from build123d import *

# Parameters (mm, degrees)
SKETCH_1_R          = 4
EXTRUDE_1_DEPTH     = 20
SKETCH_2_R          = 17
CUT_EXTRUDE_1_DEPTH = 5
CUT_EXTRUDE_START   = 15
SKETCH_2_2_R        = 17
CUT_EXTRUDE_2_DEPTH = 5


with BuildPart() as part:
    # 草图1 → 凸台-拉伸1 (new body)
    with BuildSketch(Plane.XY):
        with BuildLine():
            Line((0, 15), (75, 15))
            ThreePointArc((75, 15), (90, 0), (75, -15))
            Line((75, -15), (0, -15))
            ThreePointArc((0, -15), (-15, 0), (0, 15))
        make_face()
        Circle(SKETCH_1_R, mode=Mode.SUBTRACT)
        with Locations((75, 0)):
            Circle(SKETCH_1_R, mode=Mode.SUBTRACT)
    extrude(amount=EXTRUDE_1_DEPTH)

    # 草图2 → 切除-拉伸1 (cut)
    with BuildSketch(Plane.XY):
        Circle(SKETCH_2_R)
    extrude(amount=CUT_EXTRUDE_1_DEPTH, mode=Mode.SUBTRACT)

    # 草图2<2> → 切除-拉伸2 (cut)
    with BuildSketch(Plane.XY.offset(CUT_EXTRUDE_START)):
        Circle(SKETCH_2_2_R)
    extrude(amount=CUT_EXTRUDE_2_DEPTH, mode=Mode.SUBTRACT)


solid = part.part
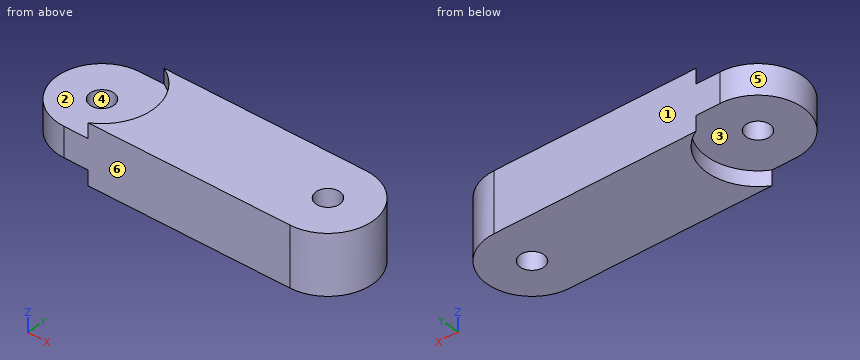
Read the model definition and answer for the solid it produces. Units are mm, in the model's axes. Face numbers are marked on the shaded views. A direction names the side the tool comes from. Give positions to 0.01 mm unless a question says otherwise; leave off trailing zeros. Loops run counter-clockwise (first coordinate to the right, second up) from the corner with the lowest first, then second, coordinate; pieces in that order, holes last. Notation, with made-up numbers: M 48,-34 L 105,-34 A15 cw 105,-5 Z; hole C 34.5,17 d5. An arc over 180 degrees is marked long. Write each question's results on one line, items separated by ' | '.
1. Section B-B on z = 3 is taken. Give the vertices of the cut face in (x, y), plus the area to 3 significant figures.
Values:
outline: M 8,-15 L 75,-15 A15 ccw 75,15 L 8,15 A17 cw Z; hole C 75,0 d8 | area: 2,120 mm^2
2. Section D-D on z = 11.75 is taken. Give the vertices of the cut face in (x, y), plus the area to 3 significant figures.
Values:
outline: M 0,-15 L 75,-15 A15 ccw 75,15 L 0,15 A15 ccw Z; hole C 0,0 d8; hole C 75,0 d8 | area: 2,860 mm^2
3. Section C-C on x = 76 is taken. Give the vertices of the cut face in (y, z).
Values:
outline: M -14.97,0 L -3.87,0 L -3.87,20 L -14.97,20 Z; M 3.87,0 L 14.97,0 L 14.97,20 L 3.87,20 Z
4. Given pin 1 (4 mm diameter, centred on x = 55.5, y = 10.5, fed in from -Z); pin 2 (9 mm diameter, centred on x = 4, y = -2, fed in from +Z); pin 3 (15 mm diameter, centred on x = -2, y = -3.5, fed in from -Z); pin 4 (8 mm diameter, centred on y = -10.5, z = 2.5, fed in from +X), each flat-ended and moving along its own axis, determine where each tip first touches the part or whether it passes through.
Values:
pin 1: stops at z = 0 | pin 2: stops at z = 15 | pin 3: stops at z = 5 | pin 4: stops at x = 88.52
5. Straight lines are drawn through the part: line 1 (Y direction, x = 75, z = 9); line 2 (Z direction, x = -9.5, y = 4); line 3 (X direction, y = 1, z = 7.5). For each, find the intervals that lie inside material, in ascending order. Write a range as [from, to].
Values:
line 1: y = [-15, -4], [4, 15] | line 2: z = [5, 15] | line 3: x = [-14.97, -3.87], [3.87, 71.13], [78.87, 89.97]
6. Section A-A on y = 0 is taken. Give the vertices of the cut face in (x, z).
Values:
outline: M -15,5 L -4,5 L -4,15 L -15,15 Z; M 4,5 L 17,5 L 17,0 L 71,0 L 71,20 L 17,20 L 17,15 L 4,15 Z; M 79,0 L 90,0 L 90,20 L 79,20 Z
7. The mould has two halves that part along Y. Classify the marked faces 4, 5 and 6: pulls with the +Y half, pulls with the -Y half, needs draft (parallel to the pull), parting line crosses it, or undercut.
Values:
face 4: undercut | face 5: parting line crosses it | face 6: pulls with the -Y half
8. A tool of negligible diameter and unlimited length cuts with its end or side. For the marked faces 1, 2 and 3, from which of +Z, -Z, +X, -X, +Y, -Y can it reach the whole face along a straight path? Write none if from no direction.
Values:
face 1: +Z, -Z, +X, -X, +Y | face 2: +Z, -X | face 3: -Z, -X
